Autodesk Inventor part; units mm, degrees
ref_plane "XZ Plane" through (0, 0, 0) normal (0, 1, 0) x (-1, 0, 0)
ref_plane "XY Plane" through (0, 0, 0) normal (0, 0, 1) x (1, 0, 0)
sketch "Sketch2" plane through (0, 0, 0) normal (0, 0, 1) x (1, 0, 0)
  line L0 (25.1049, -5.6982) -> (25.1049, -19.8714)
  arc A0 (22.4633, -22.513) -> (25.1049, -19.8714) centre (22.4633, -19.8714) ccw
  line L1 (22.4633, -22.513) -> (2.9815, -22.513)
  arc A1 (0.3399, -19.8714) -> (2.9815, -22.513) centre (2.9815, -19.8714) ccw
  line L2 (0.3399, -19.8714) -> (0.3399, -5.6982)
  arc A2 (6.3851, 0.347) -> (0.3399, -5.6982) centre (6.3851, -5.6982) ccw
  line L3 (6.3851, 0.347) -> (19.0597, 0.347)
  arc A3 (25.1049, -5.6982) -> (19.0597, 0.347) centre (19.0597, -5.6982) ccw
  line L4 (19.0597, 2.506) -> (6.3851, 2.506)
  arc A4 (6.3851, 2.506) -> (-1.8191, -5.6982) centre (6.3851, -5.6982) ccw
  line L5 (-1.8191, -5.6982) -> (-1.8191, -19.8714)
  arc A5 (-1.8191, -19.8714) -> (2.9815, -24.672) centre (2.9815, -19.8714) ccw
  line L6 (2.9815, -24.672) -> (22.4633, -24.672)
  arc A6 (22.4633, -24.672) -> (27.2639, -19.8714) centre (22.4633, -19.8714) ccw
  line L7 (27.2639, -19.8714) -> (27.2639, -5.6982)
  arc A7 (27.2639, -5.6982) -> (19.0597, 2.506) centre (19.0597, -5.6982) ccw
  line L8 (19.0597, -0.923) -> (6.3851, -0.923)
  arc A8 (6.3851, -0.923) -> (1.6099, -5.6982) centre (6.3851, -5.6982) ccw
  line L9 (1.6099, -5.6982) -> (1.6099, -19.8714)
  arc A9 (1.6099, -19.8714) -> (2.9815, -21.243) centre (2.9815, -19.8714) ccw
  line L10 (2.9815, -21.243) -> (22.4633, -21.243)
  arc A10 (22.4633, -21.243) -> (23.8349, -19.8714) centre (22.4633, -19.8714) ccw
  line L11 (23.8349, -19.8714) -> (23.8349, -5.6982)
  arc A11 (23.8349, -5.6982) -> (19.0597, -0.923) centre (19.0597, -5.6982) ccw
  point P0 (0, 0)
  dimension "d30" = 1.27
extrude "Extrusion1" add sketch "Sketch2" along normal blind 10.16 contours A7 L7 A6 L6 A5 L5 A4 L4
sketch "Sketch6" plane through (0, 0, 10.16) normal (0, 0, 1) x (1, 0, 0)
  arc A0 (22.4633, -22.513) -> (25.1049, -19.8714) centre (22.4633, -19.8714) ccw
  line L0 (22.4633, -22.513) -> (2.9815, -22.513)
  arc A1 (0.3399, -19.8714) -> (2.9815, -22.513) centre (2.9815, -19.8714) ccw
  line L1 (0.3399, -19.8714) -> (0.3399, -5.6982)
  arc A2 (6.3851, 0.347) -> (0.3399, -5.6982) centre (6.3851, -5.6982) ccw
  line L2 (6.3851, 0.347) -> (19.0597, 0.347)
  arc A3 (25.1049, -5.6982) -> (19.0597, 0.347) centre (19.0597, -5.6982) ccw
  line L3 (25.1049, -5.6982) -> (25.1049, -19.8714)
  line L4 (19.0597, 2.506) -> (6.3851, 2.506)
  arc A4 (6.3851, 2.506) -> (-1.8191, -5.6982) centre (6.3851, -5.6982) ccw
  line L5 (-1.8191, -5.6982) -> (-1.8191, -19.8714)
  arc A5 (-1.8191, -19.8714) -> (2.9815, -24.672) centre (2.9815, -19.8714) ccw
  line L6 (2.9815, -24.672) -> (22.4633, -24.672)
  arc A6 (22.4633, -24.672) -> (27.2639, -19.8714) centre (22.4633, -19.8714) ccw
  line L7 (27.2639, -19.8714) -> (27.2639, -5.6982)
  arc A7 (27.2639, -5.6982) -> (19.0597, 2.506) centre (19.0597, -5.6982) ccw
  point P0 (0, 0)
extrude "Extrusion2" add sketch "Sketch6" against normal blind 2.54 contours L0 A1 L1 A2 L2 A3 L3 A0
sketch "Sketch7" plane through (0, 0, 10.16) normal (0, 0, 1) x (1, 0, 0)
  circle A0 centre (12.7224, -11.083) radius 9.2329
  line L0 (27.2639, -19.8714) -> (27.2639, -5.6982) construction
  line L1 (19.0597, 2.506) -> (6.3851, 2.506) construction
  line L2 (2.9815, -24.672) -> (22.4633, -24.672) construction
  line L3 (-1.8191, -5.6982) -> (-1.8191, -19.8714) construction
  line L4 (10.7523, 2.506) -> (10.7523, -24.672) construction
  line L5 (-1.8191, -7.0342) -> (27.2639, -7.0342) construction
  point P0 (0, 0)
  point P1 (12.7224, -7.0342)
  point P2 (10.7523, -11.083)
  dimension "d8" = 18.4658
extrude "Extrusion3" cut sketch "Sketch7" against normal up to next
sketch "Sketch8" plane through (0, 0, 10.16) normal (0, 0, 1) x (1, 0, 0)
  circle A0 centre (12.7224, -11.083) radius 9.2329
  circle A1 centre (12.7224, -11.083) radius 9.8425
  point P0 (0, 0)
  dimension "d16" = 19.685
extrude "Extrusion4" cut sketch "Sketch8" against normal blind 1.016
sketch "Sketch9" plane through (0, 0, 10.16) normal (0, 0, 1) x (1, 0, 0)
  line L0 (11.3254, 0.1311) -> (14.1194, 0.1311)
  line L1 (14.1194, 0.1311) -> (14.1194, -3.581)
  line L2 (14.1194, -3.581) -> (11.3254, -3.581)
  line L3 (11.3254, -3.581) -> (11.3254, 0.1311)
  circle A0 centre (12.7224, -11.083) radius 9.8425
  line L4 (15.693, -1.2405) -> (10.0356, -1.2405) construction
  point P0 (0, 0)
  point P1 (12.7224, 0.1311)
  dimension "d19" = 2.794
  dimension "d21" = 1.3716
extrude "Extrusion5" cut sketch "Sketch9" against normal blind 3.175 contours L0 L1 A0 L3 | A0 L1 L2 L3 picked at (12.5667, -2.8045)
sketch "Sketch10" plane through (6.3851, 0.347, 0) normal (0, -1, 0) x (1, 0, 0)
  line L0 (12.6746, 7.62) -> (0, 7.62)
  line L1 (0, 0) -> (0, 7.62)
  line L2 (12.6746, 0) -> (0, 0)
  line L3 (12.6746, 0) -> (12.6746, 7.62)
  point P0 (-6.3851, 0)
extrude "Extrusion6" add sketch "Sketch10" along normal blind 6.35
sketch "Sketch11" plane through (6.3851, -6.003, 0) normal (-1, 0, 0) x (0, 0, 1)
  line L0 (8.0792, 4.1021) -> (0.254, -0.4699)
  line L1 (7.62, 1.6345) -> (7.62, 4.0466)
  line L2 (7.62, 1.6345) -> (7.62, 0)
  line L3 (7.62, 0) -> (7.62, 4.064)
  line L4 (7.62, 0) -> (0.762, 0)
  line L5 (0, 0) -> (7.62, 0)
  line L6 (7.62, 4.0466) -> (9.144, 4.0466)
  line L7 (0.762, 0) -> (7.62, 4.0466)
  point P0 (0, 6.003)
  dimension "d26" = 4.064
  dimension "d27" = 6.858
extrude "Extrusion7" cut sketch "Sketch11" against normal up to surface (12.6746 mm away) contours L1 L2 L4 L0 | L0 L4 L7 L1
ref_plane "Work Plane2" through (2.9815, -11.083, 0) normal (0, -1, 0) x (1, 0, 0)
mirror "Mirror1" about plane through (2.9815, -11.083, 0) normal (0, -1, 0) of "Extrusion6", "Extrusion7"
sketch "Sketch13" plane through (0, 0, 0) normal (0, 0, -1) x (-1, 0, 0)
  line L0 (-25.1049, -5.6982) -> (-25.1049, -19.8714)
  arc A0 (-25.1049, -19.8714) -> (-22.4633, -22.513) centre (-22.4633, -19.8714) ccw
  line L1 (-22.4633, -22.513) -> (-2.9815, -22.513)
  arc A1 (-2.9815, -22.513) -> (-0.3399, -19.8714) centre (-2.9815, -19.8714) ccw
  line L2 (-0.3399, -19.8714) -> (-0.3399, -5.6982)
  arc A2 (-0.3399, -5.6982) -> (-6.3851, 0.347) centre (-6.3851, -5.6982) ccw
  line L3 (-6.3851, 0.347) -> (-19.0597, 0.347)
  arc A3 (-19.0597, 0.347) -> (-25.1049, -5.6982) centre (-19.0597, -5.6982) ccw
  line L4 (-19.0597, 2.506) -> (-6.3851, 2.506)
  arc A4 (1.8191, -5.6982) -> (-6.3851, 2.506) centre (-6.3851, -5.6982) ccw
  line L5 (1.8191, -5.6982) -> (1.8191, -19.8714)
  arc A5 (-2.9815, -24.672) -> (1.8191, -19.8714) centre (-2.9815, -19.8714) ccw
  line L6 (-2.9815, -24.672) -> (-22.4633, -24.672)
  arc A6 (-27.2639, -19.8714) -> (-22.4633, -24.672) centre (-22.4633, -19.8714) ccw
  line L7 (-27.2639, -19.8714) -> (-27.2639, -5.6982)
  arc A7 (-19.0597, 2.506) -> (-27.2639, -5.6982) centre (-19.0597, -5.6982) ccw
  line L8 (-19.0597, -0.161) -> (-6.3851, -0.161)
  arc A8 (-0.8479, -5.6982) -> (-6.3851, -0.161) centre (-6.3851, -5.6982) ccw
  line L9 (-0.8479, -5.6982) -> (-0.8479, -19.8714)
  arc A9 (-2.9815, -22.005) -> (-0.8479, -19.8714) centre (-2.9815, -19.8714) ccw
  line L10 (-2.9815, -22.005) -> (-22.4633, -22.005)
  arc A10 (-24.5969, -19.8714) -> (-22.4633, -22.005) centre (-22.4633, -19.8714) ccw
  line L11 (-24.5969, -19.8714) -> (-24.5969, -5.6982)
  arc A11 (-19.0597, -0.161) -> (-24.5969, -5.6982) centre (-19.0597, -5.6982) ccw
  point P0 (0, 0)
  dimension "d32" = 0.508
extrude "Extrusion8" add sketch "Sketch13" against normal up to surface (7.62 mm away) contours A3 L3 A2 L2 A1 L1 A0 L0
sketch "Sketch14" plane through (0, 0, 10.16) normal (0, 0, 1) x (1, 0, 0)
  line L0 (19.0597, 2.506) -> (6.3851, 2.506)
  arc A0 (6.3851, 2.506) -> (-1.8191, -5.6982) centre (6.3851, -5.6982) ccw
  line L1 (-1.8191, -5.6982) -> (-1.8191, -19.8714)
  arc A1 (-1.8191, -19.8714) -> (2.9815, -24.672) centre (2.9815, -19.8714) ccw
  line L2 (2.9815, -24.672) -> (22.4633, -24.672)
  arc A2 (22.4633, -24.672) -> (27.2639, -19.8714) centre (22.4633, -19.8714) ccw
  line L3 (27.2639, -19.8714) -> (27.2639, -5.6982)
  arc A3 (27.2639, -5.6982) -> (19.0597, 2.506) centre (19.0597, -5.6982) ccw
  line L4 (11.3254, -1.3402) -> (11.3254, 0.1311)
  line L5 (11.3254, 0.1311) -> (14.1194, 0.1311)
  line L6 (14.1194, 0.1311) -> (14.1194, -1.3402)
  arc A4 (11.3254, -1.3402) -> (14.1194, -1.3402) centre (12.7224, -11.083) ccw
  line L7 (6.3851, 0.474) -> (19.0597, 0.474)
  arc A5 (25.2319, -5.6982) -> (19.0597, 0.474) centre (19.0597, -5.6982) ccw
  line L8 (25.2319, -5.6982) -> (25.2319, -19.8714)
  arc A6 (22.4633, -22.64) -> (25.2319, -19.8714) centre (22.4633, -19.8714) ccw
  line L9 (22.4633, -22.64) -> (2.9815, -22.64)
  arc A7 (0.2129, -19.8714) -> (2.9815, -22.64) centre (2.9815, -19.8714) ccw
  line L10 (0.2129, -19.8714) -> (0.2129, -5.6982)
  arc A8 (6.3851, 0.474) -> (0.2129, -5.6982) centre (6.3851, -5.6982) ccw
  arc A9 (27.2639, -5.6982) -> (19.0597, 2.506) centre (19.0597, -5.6982) ccw
  line L11 (27.2639, -19.8714) -> (27.2639, -5.6982)
  line L12 (27.2639, -5.6982) -> (25.2319, -5.6982)
  line L13 (0.2129, -5.6982) -> (-1.8191, -5.6982)
  point P0 (0, 0)
  dimension "d35" = 2.032
extrude "Extrusion9" add sketch "Sketch14" along normal blind 6.35 contours A3 L12 A5 L7 A8 L13 A0 L0
sketch "Sketch15" plane through (27.2639, -19.8714, 0) normal (1, 0, 0) x (0, 0, -1)
  line L0 (-10.16, 14.1732) -> (-16.51, 14.1732)
  line L1 (-16.51, 22.3774) -> (-16.51, 14.1732)
  arc A0 (-10.16, 14.1732) -> (-16.51, 22.3774) centre (-19.3004, 13.6582) ccw
  line L2 (-10.16, 14.1732) -> (-16.51, 14.1732)
  point P0 (0, 19.8714)
extrude "Extrusion10" cut sketch "Sketch15" against normal through all
sketch "Sketch16" plane through (0, 0, 0) normal (0, 0, -1) x (-1, 0, 0)
  line L0 (-25.1049, -5.6982) -> (-25.1049, -19.8714)
  arc A0 (-25.1049, -19.8714) -> (-22.4633, -22.513) centre (-22.4633, -19.8714) ccw
  line L1 (-22.4633, -22.513) -> (-2.9815, -22.513)
  arc A1 (-2.9815, -22.513) -> (-0.3399, -19.8714) centre (-2.9815, -19.8714) ccw
  line L2 (-0.3399, -19.8714) -> (-0.3399, -5.6982)
  arc A2 (-0.3399, -5.6982) -> (-6.3851, 0.347) centre (-6.3851, -5.6982) ccw
  line L3 (-6.3851, 0.347) -> (-19.0597, 0.347)
  arc A3 (-19.0597, 0.347) -> (-25.1049, -5.6982) centre (-19.0597, -5.6982) ccw
  line L4 (-19.0597, 2.506) -> (-6.3851, 2.506)
  arc A4 (1.8191, -5.6982) -> (-6.3851, 2.506) centre (-6.3851, -5.6982) ccw
  line L5 (1.8191, -5.6982) -> (1.8191, -19.8714)
  arc A5 (-2.9815, -24.672) -> (1.8191, -19.8714) centre (-2.9815, -19.8714) ccw
  line L6 (-2.9815, -24.672) -> (-22.4633, -24.672)
  arc A6 (-27.2639, -19.8714) -> (-22.4633, -24.672) centre (-22.4633, -19.8714) ccw
  line L7 (-27.2639, -19.8714) -> (-27.2639, -5.6982)
  arc A7 (-19.0597, 2.506) -> (-27.2639, -5.6982) centre (-19.0597, -5.6982) ccw
  line L8 (-25.9939, -5.6982) -> (-25.9939, -19.8714)
  arc A8 (-25.9939, -19.8714) -> (-22.4633, -23.402) centre (-22.4633, -19.8714) ccw
  line L9 (-22.4633, -23.402) -> (-2.9815, -23.402)
  arc A9 (-2.9815, -23.402) -> (0.5491, -19.8714) centre (-2.9815, -19.8714) ccw
  line L10 (0.5491, -19.8714) -> (0.5491, -5.6982)
  arc A10 (0.5491, -5.6982) -> (-6.3851, 1.236) centre (-6.3851, -5.6982) ccw
  line L11 (-6.3851, 1.236) -> (-19.0597, 1.236)
  arc A11 (-19.0597, 1.236) -> (-25.9939, -5.6982) centre (-19.0597, -5.6982) ccw
  point P0 (0, 0)
  dimension "d40" = 1.27
extrude "Extrusion11" cut sketch "Sketch16" against normal blind 7.62 contours L4 A4 L5 A5 L6 A6 L7 A7
sketch "Sketch17" plane through (6.3851, 1.236, 0) normal (0, 1, 0) x (1, 0, 0)
  circle A0 centre (6.3373, -3.81) radius 2.032
  line L0 (12.6746, -7.62) -> (0, -7.62)
  line L1 (0, 0) -> (0, -7.62)
  point P0 (-6.3851, 0)
  point P1 (6.3373, -7.62)
  point P2 (0, -3.81)
  dimension "d43" = 4.064
  dimension "d44" = 3.81
extrude "Extrusion12" cut sketch "Sketch17" against normal blind 6.096
mirror "Mirror2" about plane through (2.9815, -11.083, 0) normal (0, -1, 0) of "Extrusion12"
properties part number "Front"
The listing builds one solid part. Answer for the finished solid, in the listing's coordinates (mm). A direction names the side the tool comes from. Give positions to 0.01 mm unless a question says otherwise; leave off trailing zeros. Loops run counter-clockwise (first coordinate to the right, second up) from the corner with the lowest first, then second, coordinate; pieces in that order, holes last.
Item 1: A cutting plane is placed at B-B (z = 8.25). Give the vertices of the cut face in (x, y), then the cut area to 3 significant figures.
Derived:
outline: (-1.82, -19.87) arc R4.8 ccw to (2.98, -24.67) - (22.46, -24.67) arc R4.8 ccw to (27.26, -19.87) - (27.26, -5.7) arc R8.2 ccw to (19.06, 2.51) - (6.39, 2.51) arc R8.2 ccw to (-1.82, -5.7) - close; hole (11.33, -1.96) arc R9.23 ccw (long way) to (14.12, -1.96) - (14.12, 0.13) - (11.33, 0.13) - close
area: 478 mm2
Item 2: A tool of negligible diameter and unlimited length cuts with its end or side. For faces 1 (the cylindrical face through (1.489, -21.397, 3.757)), 2 (the flat face through (14.042, -3.109, 5.667)), 3 (the flat face through (13, -4.86, 2)), from which of +Z, -Z, +X, -X, +Y, -Y can it reach the whole face along a straight path? Write none if from no direction.
Derived:
face 1: -Z
face 2: none
face 3: +Z, +Y
Item 3: A cutting plane is placed at C-C (x = 12.5). Give the number of separate pieces and of enclosed holes in the cut face, then the cut area to 3 significant figures.
Derived:
separate pieces: 4
enclosed holes: 0
area: 64.4 mm2
Item 4: Determine the mould class of faces 4 (the cylindrical face through (23.99, -21.36, 3.76)), 5 (the cylindrical face through (25.895, -23.228, 8.872)), 6 (the cylindrical face through (23.91, -0.74, 3.76)) for opening direction Y: +Y half, -Y half, draft (parallel to the pull), parting line (faces both ways), or undercut.
Derived:
face 4: undercut
face 5: -Y half
face 6: +Y half
Item 5: A cutting plane is placed at A-A (x = 16.75). Give the vertices of the cut face in (y, z), then the cut area to 3 significant figures.
Derived:
outline: (-24.67, 7.62) - (-23.4, 7.62) - (-23.4, 0) - (-16.16, 0) - (-16.16, 0.76) - (-20.21, 7.62) - (-19.39, 7.62) - (-19.39, 9.14) - (-20.06, 9.14) - (-20.06, 10.16) - (-24.67, 10.16) - close; (-6, 0) - (1.24, 0) - (1.24, 7.62) - (2.51, 7.62) - (2.51, 16.51) arc R9.15 cw to (0.47, 13.05) - (0.47, 10.16) - (-2.1, 10.16) - (-2.1, 9.14) - (-2.77, 9.14) - (-2.77, 7.62) - (-1.96, 7.62) - (-6, 0.76) - close
area: 117 mm2
Item 6: Each of these flat-tipped pins is pushed along its axis until it touches: pin 1 Ø5 at (x, z) = (5, 13) entering from -Y; pin 2 Ø4 at (y, z) = (-12.5, 4) entering from -X; pin 3 Ø3 at (x, z) = (1.5, 3.5) entering from +Y. Where does it stop, or does it pass through?
Derived:
pin 1: stops at y = -0.73
pin 2: stops at x = -0.55
pin 3: stops at y = 0.35
Item 7: Find the intervals of material crossed by line 1 along X through (y, z) = (-2.5, 2); line 2 along X through (y, z) = (-2.5, 5.5); line 3 along X through (y, z) = (-7.25, 2.75), in increasing order.
Derived:
line 1: x = 0.23 to 1.86, 6.39 to 11.8, 13.65 to 19.06, 23.58 to 25.21
line 2: x = 0.23 to 1.86, 6.39 to 11.59, 13.85 to 19.06, 23.58 to 25.21
line 3: x = -0.55 to 0.85, 24.6 to 25.99
